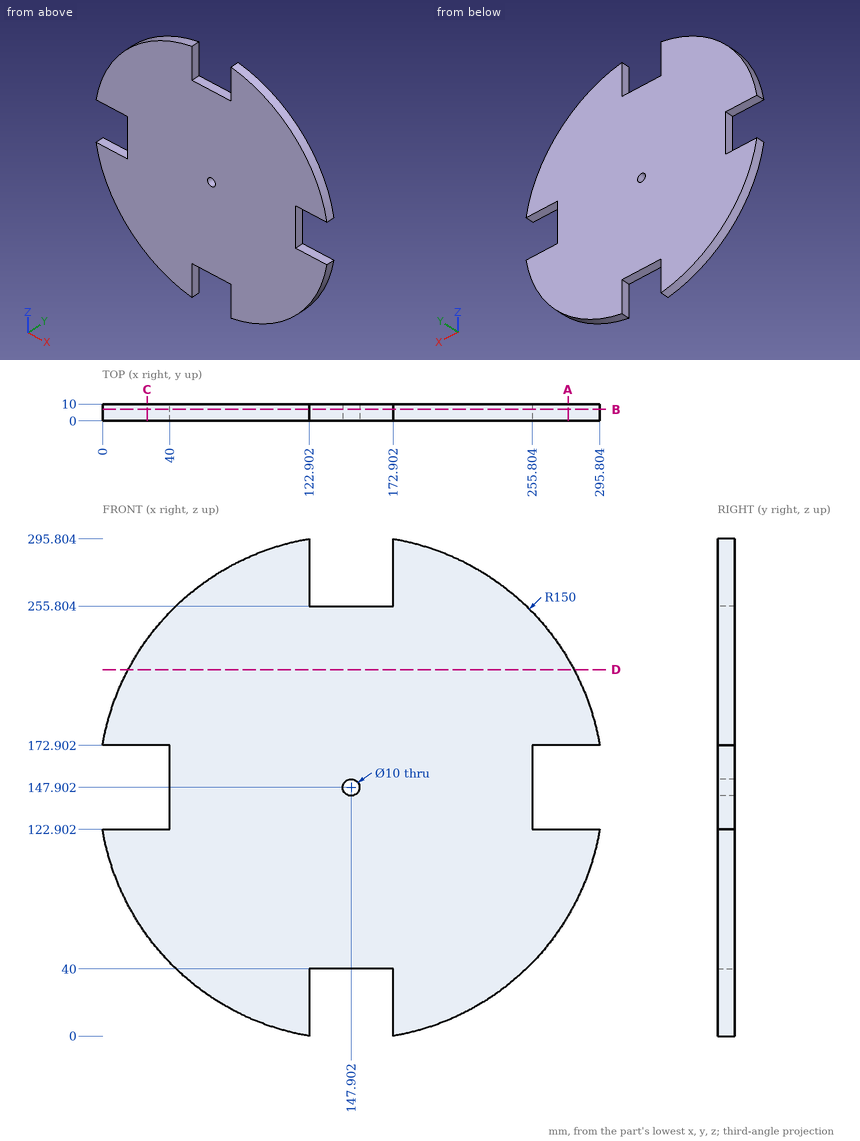
Study the drawing (mm; zero at the part's minimum x, y, z) and answer. Round coordinates to 2 decimals unless told otherwise and drop trailing zeros. Loops run counter-clockwise (first coordinate to the right, second up) from the corner with the lowest first, then second, coordinate; pieces in that order, holes last.
Q1. Section B-B, the plane y = 6.75 is taken. Determine the outline of the cut face in (x, z), then the cut area to 3 significant figures.
Q2. Given pin 1 Ø5 at (x, y) = (148.5, 3.5) entering from -Z; pin 2 Ø3 at (y, z) = (7, 272) entering from +X; pin 3 Ø1 at (x, y) = (244, 3) entering from +Z; pin 4 Ø9 at (x, z) = (147.9, 147.9) entering from +Y, each flat-ended and moving along its own axis, determine where each tip first touches the part or whether it passes through.
Q3. Section C-C, the plane x = 26.5 is taken. Determine the outline of the cut face in (y, z), then the cut area to 3 significant figures.
Q4. Section A-A, the plane x = 277 is taken. Determine the outline of the cut face in (y, z), then the cut area to 3 significant figures.
Q5. Find the intervals of material crossed by line 1 (X direction, y = 2.75, z = 148); line 2 (Z direction, x = 138.5, y = 4.75); line 3 (Z direction, x = 272, y = 3.25), in increasing order.
Q6. Section D-D, the plane z = 218 is taken. Determine the outline of the cut face in (x, y).
Completed:
1. outline: (0, 122.9) arc R150 ccw to (122.9, 0) - (122.9, 40) - (172.9, 40) - (172.9, 0) arc R150 ccw to (295.8, 122.9) - (255.8, 122.9) - (255.8, 172.9) - (295.8, 172.9) arc R150 ccw to (172.9, 295.8) - (172.9, 255.8) - (122.9, 255.8) - (122.9, 295.8) arc R150 ccw to (0, 172.9) - (40, 172.9) - (40, 122.9) - close; hole circle Ø10 at (147.9, 147.9)
1. area: 62,300 mm2
2. pin 1: stops at z = 40
2. pin 2: stops at x = 234.33
2. pin 3: stops at z = 263.49
2. pin 4: passes through
3. outline: (0, 59.8) - (10, 59.8) - (10, 122.9) - (0, 122.9) - close; (0, 172.9) - (10, 172.9) - (10, 236) - (0, 236) - close
3. area: 1,260 mm2
4. outline: (0, 71.52) - (10, 71.52) - (10, 122.9) - (0, 122.9) - close; (0, 172.9) - (10, 172.9) - (10, 224.28) - (0, 224.28) - close
4. area: 1,030 mm2
5. line 1: x = 40 to 142.9, 152.9 to 255.8
5. line 2: z = 40 to 255.8
5. line 3: z = 63.64 to 122.9, 172.9 to 232.16
6. outline: (15.29, 0) - (280.52, 0) - (280.52, 10) - (15.29, 10) - close
